from build123d import *

# Parameters (mm, degrees)
SKETCH_1_W           = 62
SKETCH_1_H           = 35
SKETCH_1_R           = 10.5
EXTRUDE_1_DEPTH      = 4
SKETCH_3_R           = 15
SKETCH_3_R_2         = 10.5
EXTRUDE_2_DEPTH      = 5
EXTRUDE_2_DEPTH_BACK = 1
FILLET_1_R           = 10
SKETCH_4_W           = 4
SKETCH_4_H           = 35
EXTRUDE_3_DEPTH      = 10
CHAMFER_1_SIZE       = 5
SKETCH_5_R           = 1.6
CUT_EXTRUDE_1_DEPTH  = 25
SKETCH_6_R           = 3
CUT_EXTRUDE_2_DEPTH  = 25
SKETCH_7_W           = 33.228870124
SKETCH_7_H           = 2.665820387
CUT_EXTRUDE_3_DEPTH  = 50
SKETCH_8_R           = 15
SKETCH_8_R_2         = 9
EXTRUDE_4_DEPTH      = 2


with BuildPart() as part:
    # Эскиз1 → Бобышка-Вытянуть1 (new body)
    with BuildSketch(Plane(origin=(0, 0, 0), x_dir=(1, 0, 0), z_dir=(0, 1, 0))):
        Rectangle(SKETCH_1_W, SKETCH_1_H)
        with Locations((-14, 0)):
            Circle(SKETCH_1_R, mode=Mode.SUBTRACT)
    extrude(amount=EXTRUDE_1_DEPTH)

    # Эскиз3 → Бобышка-Вытянуть2 (add, two sides)
    with BuildSketch(Plane(origin=(0, 0, 0), x_dir=(1, 0, 0), z_dir=(0, 1, 0))) as extrude_2_sk:
        with Locations((-14, 0)):
            Circle(SKETCH_3_R)
        with Locations((-14, 0)):
            Circle(SKETCH_3_R_2, mode=Mode.SUBTRACT)
    extrude(amount=EXTRUDE_2_DEPTH)
    extrude(extrude_2_sk.sketch, amount=-EXTRUDE_2_DEPTH_BACK)

    # Скругление1
    fillet_1_edges = [part.edges().sort_by_distance(p)[0] for p in [
        (-31, 2, -17.5),
        (-31, 2, 17.5),
    ]]
    fillet(fillet_1_edges, radius=FILLET_1_R)

    # Эскиз4 → Бобышка-Вытянуть3 (add)
    with BuildSketch(Plane(origin=(0, 4, 0), x_dir=(1, 0, 0), z_dir=(0, 1, 0))):
        with Locations((29, 0)):
            Rectangle(SKETCH_4_W, SKETCH_4_H)
    extrude(amount=EXTRUDE_3_DEPTH)

    # Фаска1
    chamfer_1_edges = [part.edges().sort_by_distance(p)[0] for p in [
        (27, 4, 0),
    ]]
    chamfer(chamfer_1_edges, length=CHAMFER_1_SIZE)

    # Эскиз5 → Вырез-Вытянуть1 (cut)
    with BuildSketch(Plane(origin=(31, 0, 0), x_dir=(0, 0, -1), z_dir=(1, 0, 0))):
        with Locations((-11.5, 10)):
            Circle(SKETCH_5_R)
        with Locations((11.5, 10)):
            Circle(SKETCH_5_R)
    extrude(amount=-CUT_EXTRUDE_1_DEPTH, mode=Mode.SUBTRACT)

    # Эскиз6 → Вырез-Вытянуть2 (cut)
    with BuildSketch(Plane.ZY.offset(-27)):
        with Locations((-11.5, 10)):
            Circle(SKETCH_6_R)
        with Locations((11.5, 10)):
            Circle(SKETCH_6_R)
    extrude(amount=CUT_EXTRUDE_2_DEPTH, mode=Mode.SUBTRACT)

    # Эскиз7 → Вырез-Вытянуть3 (cut)
    with BuildSketch(Plane.XY.offset(17.5)):
        with Locations((-14.385564938, 5.332910194)):
            Rectangle(SKETCH_7_W, SKETCH_7_H)
    extrude(amount=-CUT_EXTRUDE_3_DEPTH, mode=Mode.SUBTRACT)

    # Эскиз8 → Бобышка-Вытянуть4 (add)
    with BuildSketch(Plane.XZ.offset(1)):
        with Locations((-14, 0)):
            Circle(SKETCH_8_R)
        with Locations((-14, 0)):
            Circle(SKETCH_8_R_2, mode=Mode.SUBTRACT)
    extrude(amount=EXTRUDE_4_DEPTH)


solid = part.part
Here's how the part is built. I have some questions about the finished solid (model axes, mm). A direction names the side the tool comes from. Round coordinates to 2 decimals unless told otherwise and drop trailing zeros. Loops run counter-clockwise (first coordinate to the right, second up) from the corner with the lowest first, then second, coordinate; pieces in that order, holes last. Notation, with made-up numbers: (60.25, 62) -> (64.25, 62) arc R16 ccw to (64.25, 66) -> close; hole circle Ø3 at (61.25, 60). An arc over 180 degrees is marked (long way). Write each question's results on one line, items separated by ' | '.
(1) We'd pull the mould along Z, two halves only. Please class faces 1 (the face through (-5.416, -1.986, 2.703)), 2 (the face through (-31, 2, 0)), 3 (the face through (-28.15, 2.03, 14.49)): released by +Z, released by -Z, zero draft, split by the parting line, or undercut.
Worked answers:
face 1: undercut | face 2: zero draft | face 3: released by +Z
(2) For P1, Ø17, axis at x = -12, z = -3.5, coming from the +Y side; P2, Ø5, axis at y = 10, z = -11.5, coming from the -X side; P3, Ø3, axis at x = 7, z = -13.5, coming from the -Y side, each with a flat end and sliding along its axis, tell me the tip position at first contact or that it passes through.
Worked answers:
P1: y = 4 | P2: x = 27 | P3: y = 0
(3) If we section it at C-C, the plane y = 10: List the corners of the cut face in (x, z) for me, then the cut area to 3 significant figures.
Worked answers:
outline: (27, -17.5) -> (31, -17.5) -> (31, -13.1) -> (27, -13.1) -> close; (27, -9.9) -> (31, -9.9) -> (31, 9.9) -> (27, 9.9) -> close; (27, 13.1) -> (31, 13.1) -> (31, 17.5) -> (27, 17.5) -> close | area: 114 mm2
(4) If we section it at A-A, the plane x = -14: List the corners of the cut face in (y, z) for me, then the cut area to 3 significant figures.
Worked answers:
outline: (-3, -15) -> (0, -15) -> (0, -17.5) -> (4, -17.5) -> (4, -10.5) -> (-1, -10.5) -> (-1, -9) -> (-3, -9) -> close; (-3, 9) -> (-1, 9) -> (-1, 10.5) -> (4, 10.5) -> (4, 17.5) -> (0, 17.5) -> (0, 15) -> (-3, 15) -> close | area: 89.0 mm2
(5) If we section it at B-B, the plane z = 0: List the corners of the cut face in (x, y) for me, then the cut area to 4 significant figures.
Worked answers:
outline: (-31, 0) -> (-29, 0) -> (-29, -3) -> (-23, -3) -> (-23, -1) -> (-24.5, -1) -> (-24.5, 4) -> (-31, 4) -> close; (-5, -3) -> (1, -3) -> (1, 0) -> (31, 0) -> (31, 14) -> (27, 14) -> (27, 9) -> (22, 4) -> (-3.5, 4) -> (-3.5, -1) -> (-5, -1) -> close | area: 249.5 mm2
(6) If I drill on L1, parallel to X at y = 0.65, z = 0; L2, parallel to Z at x = -14, y = -1.6; L3, parallel to Z at x = -14, y = 2.55, over which ranges is the centre line in solid material (lowest first)?
Worked answers:
L1: -31 to -24.5, -3.5 to 31 | L2: -15 to -9, 9 to 15 | L3: -17.5 to -10.5, 10.5 to 17.5
(7) For faces 4 (the face through (26.1, 7, 11.4)), 5 (the face through (1, 4, 0)), 6 (the face through (-4, 1.5, -3.2)), 7 (the face through (10.4, 3.8, -17.5)), 8 (the face through (-28.985, -1.479, 0.66)), which set-ups out of +Z, -Z, +X, -X, +Y, -Y let a thin tool reach every point of the face, with its end or its side?
Worked answers:
face 4: -X, +Y | face 5: +Z, -Z, -X, +Y | face 6: +Y | face 7: -Z, +X, -X, +Y, -Y | face 8: -Y
(8) If we section it at D-D, the plane y = 3.25: List the corners of the cut face in (x, z) for me.
Worked answers:
outline: (-31, -7.5) arc R10 ccw to (-21, -17.5) -> (31, -17.5) -> (31, 17.5) -> (-21, 17.5) arc R10 ccw to (-31, 7.5) -> close; hole circle Ø21 at (-14, 0)
